```python
from build123d import *

# Parameters (mm, degrees)
EXTRUDE_1_DEPTH     = 2
SKETCH_2_W          = 6
SKETCH_2_H          = 35
EXTRUDE_2_DEPTH     = 60
FILLET_1_R          = 17.5
SKETCH_3_R          = 16
CUT_EXTRUDE_1_DEPTH = 5
CHAMFER_1_SIZE      = 1.640243073
CHAMFER_1_SIZE_2    = 0.8
SKETCH_4_R          = 15
CUT_EXTRUDE_2_DEPTH = 105.385422037
SKETCH_5_W          = 25
SKETCH_5_H          = 10.5
EXTRUDE_3_DEPTH     = 7.3
EXTRUDE_4_DEPTH     = 2
FILLET_2_R          = 1
EXTRUDE_5_DEPTH     = 5
SKETCH_9_R          = 1.15
CUT_EXTRUDE_3_DEPTH = 101.277297201
SKETCH_10_R         = 2
CUT_EXTRUDE_4_DEPTH = 10
FILLET_3_R          = 0.5
SKETCH_12_W         = 56.21
SKETCH_12_H         = 29.03
CUT_EXTRUDE_5_DEPTH = 113.159332301
BOSS_EXTRUDE1_DEPTH = 6
BOSS_EXTRUDE2_DEPTH = 0.5
BOSS_EXTRUDE3_DEPTH = 0.5
SKETCH5_W           = 0.5
SKETCH5_H           = 2
BOSS_EXTRUDE4_DEPTH = 2
CUT_EXTRUDE1_DEPTH  = 9
SKETCH6_W           = 1
SKETCH6_H           = 9.3
BOSS_EXTRUDE5_DEPTH = 2
SKETCH7_W           = 1
SKETCH7_H           = 9.3
BOSS_EXTRUDE7_DEPTH = 3
FILLET1_R           = 1


# Some blends are built 0.0001 mm under size
with BuildPart() as part:
    # 스케치1 → 보스-돌출1 (new body)
    with BuildSketch(Plane(origin=(0, 0, 0), x_dir=(1, 0, 0), z_dir=(0, 1, 0))):
        with BuildLine():
            Line((-11.24267666, -2.527135016), (-67.45267666, -2.527135016))
            ThreePointArc((-67.45267666, -2.527135016), (-50.72671765, -44.531450868), (-11.24267666, -66.557135016))
            Line((-11.24267666, -66.557135016), (-11.24267666, -2.527135016))
        make_face()
    extrude(amount=EXTRUDE_1_DEPTH)

    # 스케치2 → 보스-돌출2 (add)
    with BuildSketch(Plane(origin=(0, 2, 0), x_dir=(1, 0, 0), z_dir=(0, 1, 0))):
        with Locations((-14.24267666, -20.027135016)):
            Rectangle(SKETCH_2_W, SKETCH_2_H)
    extrude(amount=EXTRUDE_2_DEPTH)

    # 필렛1
    fillet_1_edges = [part.edges().sort_by_distance(p)[0] for p in [
        (-14.24267666, 62, 2.527135016),
        (-14.24267666, 62, 37.527135016),
    ]]
    fillet(fillet_1_edges, radius=FILLET_1_R - 0.0001)  # a hair under: the kernel refuses the full size

    # 스케치3 → 컷-돌출1 (cut)
    with BuildSketch(Plane(origin=(-11.24267666, 0, 0), x_dir=(0, 0, -1), z_dir=(1, 0, 0))):
        with Locations((-20.027135016, 44.5)):
            Circle(SKETCH_3_R)
    extrude(amount=-CUT_EXTRUDE_1_DEPTH, mode=Mode.SUBTRACT)

    # 모따기1
    # the kernel refuses this chamfer: 1.640243073, 0.8 mm, written as the material it takes off along each edge
    with BuildSketch(Plane(origin=(-11.24267666, 44.5, 20.027135016), x_dir=(0, 0, -1), z_dir=(0, -1, 0))) as chamfer_1_piece_1:
        Polygon((16 + CHAMFER_1_SIZE, 0), (16, -CHAMFER_1_SIZE_2), (16, 0), align=None)
    revolve(axis=Axis((-11.24267666, 44.5, 20.027135016), (1, 0, 0)), mode=Mode.SUBTRACT)

    # 스케치4 → 컷-돌출2 (cut, through all)
    with BuildSketch(Plane(origin=(-16.24267666, 0, 0), x_dir=(0, 0, -1), z_dir=(1, 0, 0))):
        with Locations((-20.027135016, 44.5)):
            Circle(SKETCH_4_R)
    extrude(amount=-CUT_EXTRUDE_2_DEPTH, mode=Mode.SUBTRACT)

    # 스케치5 → 보스-돌출3 (add)
    with BuildSketch(Plane(origin=(0, 2, 0), x_dir=(1, 0, 0), z_dir=(0, 1, 0))):
        with Locations((-32.74267666, -7.777135016)):
            Rectangle(SKETCH_5_W, SKETCH_5_H)
        with Locations((-32.74267666, -32.277135016)):
            Rectangle(SKETCH_5_W, SKETCH_5_H)
    extrude(amount=EXTRUDE_3_DEPTH)

    # 스케치6 → 보스-돌출4 (add)
    with BuildSketch(Plane(origin=(0, 9.3, 0), x_dir=(1, 0, 0), z_dir=(0, 1, 0))):
        Polygon((-45.24267666, -32.527135016), (-25.24267666, -32.527135016), (-25.24267666, -27.027135016), (-20.24267666, -27.027135016), (-20.24267666, -37.527135016), (-45.24267666, -37.527135016), align=None)
        Polygon((-45.24267666, -2.527135016), (-20.24267666, -2.527135016), (-20.24267666, -13.027135016), (-25.24267666, -13.027135016), (-25.24267666, -7.527135016), (-45.24267666, -7.527135016), align=None)
    extrude(amount=EXTRUDE_4_DEPTH)

    # 필렛2
    fillet_2_edges = [part.edges().sort_by_distance(p)[0] for p in [
        (-45.24267666, 6.65, 2.527135016),
        (-45.24267666, 5.65, 13.027135016),
        (-45.24267666, 5.65, 27.027135016),
        (-45.24267666, 6.65, 37.527135016),
    ]]
    fillet(fillet_2_edges, radius=FILLET_2_R)

    # 스케치7 → 보스-돌출5 (add)
    with BuildSketch(Plane.ZY.offset(25.24267666)):
        with BuildLine():
            Line((2.527135016, 11.3), (13.027135016, 11.3))
            Line((13.027135016, 11.3), (13.027135016, 36.014718626))
            ThreePointArc((13.027135016, 36.014718626), (10.875170651, 38.397414624), (9.502877322, 41.3))
            Line((9.502877322, 41.3), (2.527135016, 41.3))
            Line((2.527135016, 41.3), (2.527135016, 11.3))
        make_face()
        with BuildLine():
            Line((37.527135016, 11.3), (27.027135016, 11.3))
            Line((27.027135016, 11.3), (27.027135016, 36.014718626))
            ThreePointArc((27.027135016, 36.014718626), (29.17909938, 38.397414624), (30.551392709, 41.3))
            Line((30.551392709, 41.3), (37.527135016, 41.3))
            Line((37.527135016, 41.3), (37.527135016, 11.3))
        make_face()
    extrude(amount=-EXTRUDE_5_DEPTH)

    # 스케치9 → 컷-돌출3 (cut, through all)
    with BuildSketch(Plane.ZY.offset(25.24267666)):
        with Locations((9.777135016, 35.8)):
            Circle(SKETCH_9_R)
        with Locations((9.777135016, 15.3)):
            Circle(SKETCH_9_R)
        with Locations((30.277135016, 15.3)):
            Circle(SKETCH_9_R)
        with Locations((30.277135016, 35.8)):
            Circle(SKETCH_9_R)
    extrude(amount=-CUT_EXTRUDE_3_DEPTH, mode=Mode.SUBTRACT)

    # 스케치10 → 컷-돌출4 (cut)
    with BuildSketch(Plane(origin=(-11.24267666, 0, 0), x_dir=(0, 0, -1), z_dir=(1, 0, 0))):
        with Locations((-30.277135016, 15.3)):
            Circle(SKETCH_10_R)
        with Locations((-9.777135016, 15.3)):
            Circle(SKETCH_10_R)
        with Locations((-9.777135016, 35.8)):
            Circle(SKETCH_10_R)
        with Locations((-30.277135016, 35.8)):
            Circle(SKETCH_10_R)
    extrude(amount=-CUT_EXTRUDE_4_DEPTH, mode=Mode.SUBTRACT)

    # 필렛3
    fillet_3_edges = [part.edges().sort_by_distance(p)[0] for p in [
        (-45.24267666, 10.3, 32.527135016),
        (-25.24267666, 22.657359313, 27.027135016),
        (-35.24267666, 9.3, 32.527135016),
        (-45.24267666, 9.3, 30.277135016),
        (-44.949783441, 9.3, 27.320028235),
        (-34.74267666, 9.3, 13.027135016),
        (-44.949783441, 9.3, 12.734241797),
        (-45.24267666, 9.3, 9.777135016),
        (-35.24267666, 9.3, 7.527135016),
        (-45.24267666, 10.3, 7.527135016),
        (-25.24267666, 22.657359313, 13.027135016),
        (-34.74267666, 9.3, 27.027135016),
    ]]
    fillet(fillet_3_edges, radius=FILLET_3_R)

    # 스케치12 → 컷-돌출5 (cut, through all)
    with BuildSketch(Plane(origin=(0, 2, 0), x_dir=(1, 0, 0), z_dir=(0, 1, 0))):
        with Locations((-39.34767666, -52.042135016)):
            Rectangle(SKETCH_12_W, SKETCH_12_H)
    extrude(amount=-CUT_EXTRUDE_5_DEPTH, mode=Mode.SUBTRACT)

    # Sketch1 → Boss-Extrude1 (add)
    with BuildSketch(Plane(origin=(-11.24267666, 0, 0), x_dir=(0, 0, -1), z_dir=(1, 0, 0))):
        with BuildLine():
            Line((-38.027135016, 42.280050522), (-38.027135016, 0))
            Line((-38.027135016, 0), (-37.527135016, 0))
            Line((-37.527135016, 0), (-37.527135016, 44.5))
            ThreePointArc((-37.527135016, 44.5), (-32.401503687, 56.874368671), (-20.027135016, 62))
            ThreePointArc((-20.027135016, 62), (-7.652766345, 56.874368671), (-2.527135016, 44.5))
            Line((-2.527135016, 44.5), (-2.527135016, 0))
            Line((-2.527135016, 0), (-2.027135016, 0))
            Line((-2.027135016, 0), (-2.027135016, 42.280050522))
            Line((-2.027135016, 42.280050522), (-2.027135016, 44.5))
            ThreePointArc((-2.027135016, 44.5), (-7.299212954, 57.227922061), (-20.027135016, 62.5))
            ThreePointArc((-20.027135016, 62.5), (-32.755057077, 57.227922061), (-38.027135016, 44.5))
            Line((-38.027135016, 44.5), (-38.027135016, 42.280050522))
        make_face()
    extrude(amount=-BOSS_EXTRUDE1_DEPTH)

    # Sketch2 → Boss-Extrude2 (add)
    with BuildSketch(Plane(origin=(0, 0, 2.527135016), x_dir=(-1, 0, 0), z_dir=(0, 0, -1))):
        Polygon((17.24267666, 2), (17.24267666, 0), (67.45267666, 0), (67.45267666, 2), (44.24267666, 2), (44.24267666, 11.3), (25.24267666, 11.3), (25.24267666, 41.3), (20.24267666, 41.3), (20.24267666, 2), align=None)
    extrude(amount=BOSS_EXTRUDE2_DEPTH)

    # Sketch3 → Boss-Extrude3 (add)
    with BuildSketch(Plane.XY.offset(37.527135016)):
        Polygon((-17.24267666, 0), (-17.24267666, 2), (-20.24267666, 2), (-20.24267666, 41.3), (-25.24267666, 41.3), (-25.24267666, 11.3), (-44.24267666, 11.3), (-44.24267666, 2), (-56.106720966, 2), (-56.106720966, 0), align=None)
    extrude(amount=BOSS_EXTRUDE3_DEPTH)

    # Sketch5 → Boss-Extrude4 (add)
    with BuildSketch(Plane.ZY.offset(67.45267666)):
        with Locations((2.277135016, 1)):
            Rectangle(SKETCH5_W, SKETCH5_H)
    extrude(amount=BOSS_EXTRUDE4_DEPTH)

    # Sketch4 → Cut-Extrude1 (cut)
    with BuildSketch(Plane.XZ):
        with BuildLine():
            Line((-67.498191683, 0.494084527), (-93.58337569, -4.753226021))
            Line((-93.58337569, -4.753226021), (-77.452778633, 44.072890783))
            Line((-77.452778633, 44.072890783), (-53.718589474, 40.872523105))
            ThreePointArc((-53.718589474, 40.872523105), (-63.882560875, 21.800651733), (-67.498191683, 0.494084527))
        make_face()
    extrude(amount=-CUT_EXTRUDE1_DEPTH, mode=Mode.SUBTRACT)

    # Sketch6 → Boss-Extrude5 (add)
    with BuildSketch(Plane.XY.offset(38.027135016)):
        with Locations((-44.74267666, 6.65)):
            Rectangle(SKETCH6_W, SKETCH6_H)
    extrude(amount=-BOSS_EXTRUDE5_DEPTH)

    # Sketch7 → Boss-Extrude7 (add)
    with BuildSketch(Plane(origin=(0, 0, 2.027135016), x_dir=(-1, 0, 0), z_dir=(0, 0, -1))):
        with Locations((44.74267666, 6.65)):
            Rectangle(SKETCH7_W, SKETCH7_H)
    extrude(amount=-BOSS_EXTRUDE7_DEPTH)

    # Fillet1
    fillet1_edges = [part.edges().sort_by_distance(p)[0] for p in [
        (-45.24267666, 6.65, 38.027135016),
        (-45.24267666, 6.65, 2.027135016),
    ]]
    fillet(fillet1_edges, radius=FILLET1_R)


solid = part.part
```
Check sheet for the modelled part. Datum: model origin and axes. Units: mm. A direction names the side the tool comes from. Round coordinates to 2 decimals unless told otherwise and drop trailing zeros. Loops run counter-clockwise (first coordinate to the right, second up) from the corner with the lowest first, then second, coordinate; pieces in that order, holes last. Notation, with made-up numbers: (29.5, 60) -> (73.5, 60) arc R9 cw to (73.5, 73) -> close; hole circle Ø1 at (39.25, -34.5). An arc over 180 degrees is marked (long way). Write item = value, one per line. Start each with the question number.
1) Sectioned sample at C-C, the plane x = -19.5. Record the cut outline in (y, z), plus the area to 3 significant figures.
2) Gauge pin test, flat ends, axial feed: pin 1 Ø4 at (x, z) = (-50.5, 31) entering from -Y; pin 2 Ø2 at (y, z) = (35, 9) entering from +X; pin 3 Ø2 at (x, z) = (-52, 27.5) entering from +Y; pin 4 Ø3.5 at (x, z) = (-30.5, 30.5) entering from +Y. Record the tip position at first contact, or that the pin passes through.
3) Sectioned sample at B-B, the plane x = -26.5. Record the cut outline in (y, z).
4) Release check for a two-part mould opening along Z. For faces 1 (the flat face through (-35, 11.3, 5)), 2 (the cylindrical face through (-22.778, 38.36, 29.154)), 3 (the cylindrical face through (-23.27, 14.28, 10.31)) record: released by +Z, released by -Z, zero draft, split by the parting line, or undercut.
5) Sectioned sample at A-A, the plane y = 21. Record the cut outline in (x, z), plus the area to 3 significant figures.
6) Set-up check for faces 4 (the flat face through (-16.243, 59, 15)), 5 (the flat face through (-35, 11, 7.527)), 6 (the flat face through (-23, 41.3, 6)): record each of +Z, -Z, +X, -X, +Y, -Y from which the full face is reachable in a straight line by a thin tool's end or side.
7) Thickness scan on probe 1 along Z at (x, y) = (-43.5, 4); probe 2 along Y at (x, z) = (-47.5, 33.5); probe 3 along Y at (x, z) = (-33.5, 28). Record the ranges inside material, lowest first.
Results are:
q1.outline = (0, 2.03) -> (2, 2.03) -> (2, 38.03) -> (0, 38.03) -> close
q1.area = 72.0 mm^2
q2.pin_1 = 0
q2.pin_2 = -16.24
q2.pin_3 = 2
q2.pin_4 = 9.35
q3.outline = (0, 2.03) -> (11.3, 2.03) -> (11.3, 7.53) -> (9.8, 7.53) arc R0.5 cw to (9.3, 8.03) -> (9.3, 12.53) arc R0.5 ccw to (8.8, 13.03) -> (2, 13.03) -> (2, 27.03) -> (8.8, 27.03) arc R0.5 ccw to (9.3, 27.53) -> (9.3, 32.03) arc R0.5 cw to (9.8, 32.53) -> (11.3, 32.53) -> (11.3, 38.03) -> (0, 38.03) -> close
q4.face_1 = zero draft
q4.face_2 = undercut
q4.face_3 = undercut
q5.outline = (-25.24, 2.03) -> (-20.24, 2.03) -> (-20.24, 13.03) -> (-24.74, 13.03) arc R0.5 ccw to (-25.24, 12.53) -> close; (-25.24, 27.53) arc R0.5 ccw to (-24.74, 27.03) -> (-20.24, 27.03) -> (-20.24, 38.03) -> (-25.24, 38.03) -> close; (-17.24, 2.03) -> (-11.24, 2.03) -> (-11.24, 38.03) -> (-17.24, 38.03) -> close
q5.area = 326 mm^2
q6.face_4 = +X
q6.face_5 = -X, +Y
q6.face_6 = +Z, -Z, -X, +Y
q7.probe_1 = 2.03 to 13.03, 27.03 to 38.03
q7.probe_2 = 0 to 2
q7.probe_3 = 0 to 9.3
